Input: part model. Units: mm. Frame: model coordinates. A direction names the side the tool comes from. Round coordinates to 2 decimals unless told otherwise and drop trailing zeros. Order: outer loops, then holes, each group sorted by start corner. A loop starts at its lowest first (then second) coordinate and runs counter-clockwise, first axis right, second up. Notation, with made-up numbers: (55, 34) -> (69, 34) arc R20 ccw to (69, 54) -> close; hole circle Ø5 at (-28, 64). An arc over 180 degrees is marked (long way). Use a Markdown table: item, result.
from build123d import *

# Parameters (mm, degrees)
SKETCH_1_R               = 5
EXTRUDE_1_DEPTH          = 84
SKETCH_6_W               = 79
SKETCH_6_H               = 8.752302232
CUT_EXTRUDE_1_DEPTH      = 6
CUT_EXTRUDE_1_DEPTH_BACK = 6


with BuildPart() as part:
    # Эскиз1 → Бобышка-Вытянуть1 (new body)
    with BuildSketch(Plane(origin=(0, 0, 0), x_dir=(0, 0, -1), z_dir=(1, 0, 0))):
        Circle(SKETCH_1_R)
    extrude(amount=EXTRUDE_1_DEPTH)

    # Эскиз2 → Отверстие обработанное метчиком M31 (revolve, cut)
    with BuildSketch(Plane.ZX):
        Polygon((0, 0), (0, 12.751075774), (1.25, 12), (1.25, 9), (1.5, 9), (1.5, 0.1), (1.6, 0), align=None)
    revolve(axis=Axis((-6.35, 0, 0), (1, 0, 0)), mode=Mode.SUBTRACT)

    # Эскиз4 → Отверстие обработанное метчиком M32 (revolve, cut)
    with BuildSketch(Plane(origin=(84, 0, 0), x_dir=(0, 0, -1), z_dir=(0, 1, 0))):
        Polygon((0, 0), (0, 12.751075774), (1.25, 12), (1.25, 9), (1.5, 9), (1.5, 0.1), (1.6, 0), align=None)
    revolve(axis=Axis((90.35, 0, 0), (-1, 0, 0)), mode=Mode.SUBTRACT)

    # Эскиз6 → Вырез-Вытянуть1 (cut, two sides)
    with BuildSketch(Plane(origin=(0, 0, 0), x_dir=(1, 0, 0), z_dir=(0, 1, 0))) as cut_extrude_1_sk:
        with Locations((42, 6.876151116)):
            Rectangle(SKETCH_6_W, SKETCH_6_H)
    extrude(amount=CUT_EXTRUDE_1_DEPTH, mode=Mode.SUBTRACT)
    extrude(cut_extrude_1_sk.sketch, amount=-CUT_EXTRUDE_1_DEPTH_BACK, mode=Mode.SUBTRACT)


solid = part.part
1) Contact query for flat-ended pins moving along their axis: P1, Ø1, axis at x = 23.5, z = 1, coming from the +Y side; P2, Ø1.5, axis at y = -0.5, z = -0.5, coming from the +X side; P3, Ø1, axis at x = 61, y = -2, coming from the -Z side. Output: stop coordinate, or through.
Answer key:
| item | result |
|---|---|
| P1 | stops at y = 4.97 |
| P2 | stops at x = 75 |
| P3 | stops at z = -2.5 |
2) Ray query, probe 1 along Y at (x, z) = (5.75, 0); probe 2 along X at (y, z) = (1.75, -3.25); probe 3 along Y at (x, z) = (69.5, -0.25). Return the intervals inside material, ascending.
Answer key:
| item | result |
|---|---|
| probe 1 | y = -5 to -1.5, 1.5 to 5 |
| probe 2 | x = 0 to 2.5, 81.5 to 84 |
| probe 3 | y = -4.99 to 4.99 |
3) Draft query along Y for faces 1 (the face through (2.5, 0, -3)), 2 (the face through (41, -3, 4)), 3 (the face through (4.49, -0.07, -1.5)). Return one class per face: released by +Y, released by -Y, zero draft, split by the parting line, or undercut.
Answer key:
| item | result |
|---|---|
| face 1 | zero draft |
| face 2 | split by the parting line |
| face 3 | undercut |
4) Cut plane B-B on x = 45. Return loops of the section in (y, z), and give its area (3 significant figures).
Answer key:
| item | result |
|---|---|
| outline | (-4.33, -2.5) -> (4.33, -2.5) arc R5 ccw (long way) to start |
| area | 63.2 mm^2 |
5) Cut plane C-C on y = 3.5. Return loops of the section in (x, z).
Answer key:
| item | result |
|---|---|
| outline | (0, -3.57) -> (2.5, -3.57) -> (2.5, -2.5) -> (81.5, -2.5) -> (81.5, -3.57) -> (84, -3.57) -> (84, 3.57) -> (0, 3.57) -> close |
6) Set-up query: faces 4 (the face through (79.51, -0.07, 1.5)), 5 (the face through (41, 0, -2.5)), 6 (the face through (10.48, 1.22, -0.27)). Return all of +Z, -Z, +X, -X, +Y, -Y with unobstructed straight access to the full face (end or side cutting, diameter ignored); none if empty.
Answer key:
| item | result |
|---|---|
| face 4 | +X |
| face 5 | -Z, +Y, -Y |
| face 6 | -X |
7) Cut plane A-A on z = -3.5. Return loops of the section in (x, y), and give its area (3 significant figures).
Answer key:
| item | result |
|---|---|
| outline | (0, -3.57) -> (2.5, -3.57) -> (2.5, 3.57) -> (0, 3.57) -> close; (81.5, -3.57) -> (84, -3.57) -> (84, 3.57) -> (81.5, 3.57) -> close |
| area | 35.7 mm^2 |
